Part model, mm, in its own coordinate system. Face numbers are marked on the shaded views. Round coordinates to 2 decimals unless told otherwise and drop trailing zeros. Order: outer loops, then holes, each group sorted by start corner. A loop starts at its lowest first (then second) coordinate and runs counter-clockwise, first axis right, second up. Notation, with made-up numbers: (-14, -19.75) -> (40, -19.75) arc R21 ccw to (40, 18.25) -> close; hole circle Ø3 at (15.25, -13.5). An arc over 180 degrees is marked (long way). Answer as a JSON object with one key per item and string values. Group by question number.
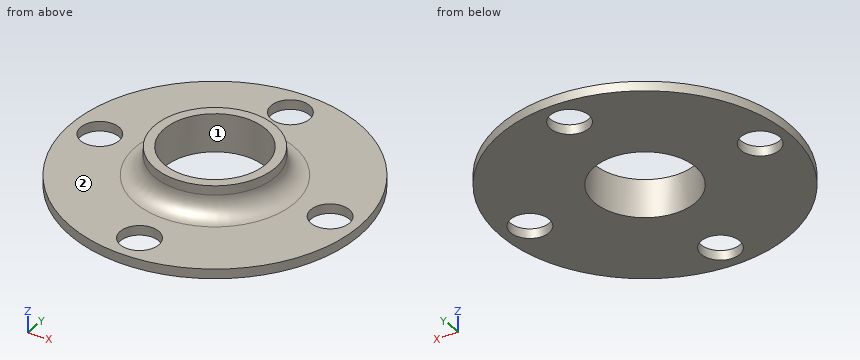
```python
from build123d import *

# Parameters (mm, degrees)
F0_R     = 47.625
F0_R_2   = 16.7005
F1_DEPTH = 12.5984
F4_R     = 6.35
F5_DEPTH = 12.5994


with BuildPart() as f1:
    # F0 (on Top) → F1 (new body)
    with BuildSketch(Plane.XY):
        Circle(F0_R)
        Circle(F0_R_2, mode=Mode.SUBTRACT)
    extrude(amount=F1_DEPTH)

    # F2 (on Front) → F3 (revolve, cut)
    with BuildSketch(Plane.XZ):
        with BuildLine():
            Line((50.8, 3.175), (50.8, 12.5984))
            Line((50.8, 12.5984), (19.8755, 12.5984))
            Line((19.8755, 12.5984), (19.8755, 9.525))
            ThreePointArc((19.8755, 9.525), (21.735372, 5.034872), (26.2255, 3.175))
            Line((26.2255, 3.175), (50.8, 3.175))
        make_face()
    revolve(axis=Axis((0, 0, 6.2992), (0, 0, 1)), mode=Mode.SUBTRACT)

    # F4 (on face) → F5 (cut, through all)
    with BuildSketch(Plane(origin=(0, 0, 0), x_dir=(1, 0, 0), z_dir=(0, 0, -1))):
        with Locations((0, 38.1)):
            Circle(F4_R)
        with Locations((0, -38.1)):
            Circle(F4_R)
        with Locations((-38.1, 0)):
            Circle(F4_R)
        with Locations((38.1, 0)):
            Circle(F4_R)
    extrude(amount=-F5_DEPTH, mode=Mode.SUBTRACT)


solid = f1.part
```
Q1. Two-plate mould, pull along X, no slides. Class the marked faces 1 and 2: +X half, -X half, draft (parallel to the pull), parting line (faces both ways), or undercut.
Q2. Drop flat-ended pins along their axis: pin 1 Ø11.5 at (x, y) = (38.1, 0) entering from -Z; pin 2 Ø5 at (x, z) = (30, 4.5) entering from -Y; pin 3 Ø6 at (y, z) = (10, 2.5) entering from +X; pin 4 Ø12 at (x, y) = (-17, -30) entering from +Z (3 decimals). Give the stop position or say it passes through.
Q3. Band-saw the part on A-A (y = 0). Count the separate pieces of the cut face and the enclosed holes in it, plus the area to 3 significant figures.
Q4. Wall check: line 1 (Y direction, x = -0.5, z = 2.75); line 2 (Z direction, x = -18, y = -33.5) (3 decimals); line 3 (X direction, y = -38.1, z = 1.45) (3 decimals). Give the ranges that are in metal, low to high. Write a range as [from, to].
Q5. Band-saw the part on D-D (x = 38.1). List the corners of the cut face in (y, z) (3 decimals).
Completed:
{
 "1": {"face 1": "undercut", "face 2": "draft"},
 "2": {"pin 1": "through", "pin 2": "y = -38.61", "pin 3": "x = 47.11", "pin 4": "z = 3.175"},
 "3": {"separate pieces": "4", "enclosed holes": "0", "area": "193 mm2"},
 "4": {"line 1": "[-47.62, -44.43], [-31.77, -16.69], [16.69, 31.77], [44.43, 47.62]", "line 2": "[0, 3.175]", "line 3": "[-28.575, -6.35], [6.35, 28.575]"},
 "5": {"outline": "(-28.575, 0) -> (-6.35, 0) -> (-6.35, 3.175) -> (-28.575, 3.175) -> close; (6.35, 0) -> (28.575, 0) -> (28.575, 3.175) -> (6.35, 3.175) -> close"}
}
